from build123d import *

# Parameters (mm, degrees)
F1_DEPTH = 800
F2_R     = 10
F3_R     = 0.2


with BuildPart() as f1:
    # F0 (on Right) → F1 (new body)
    with BuildSketch(Plane.YZ):
        Polygon((100.824344, 4.7625), (125.181556, 0), (150, 0), (2.787639, 28.784037), (1.873746, 24.110044), (6.636246, 23.178845), align=None)
        Polygon((0, 4.7625), (0, 0), (125.181556, 0), (100.824344, 4.7625), (6.636246, 4.7625), (1.873746, 4.7625), align=None)
        Polygon((1.873746, 24.110044), (1.873746, 4.7625), (6.636246, 4.7625), (6.636246, 23.178845), align=None)
        Polygon((1.873746, 24.110044), (2.787639, 28.784037), (-8.682065, 26.173362), (-5.835444, 22.355227), align=None)
        Polygon((-10.756327, 4.761424), (0, 0), (0, 4.7625), (-7.229277, 7.963836), align=None)
        Polygon((-14.458972, 15.926554), (-10.756327, 4.761424), (-7.229277, 7.963836), (-9.718587, 15.468123), align=None)
        Polygon((-8.682065, 26.173362), (-14.458972, 15.926554), (-9.718587, 15.468123), (-5.835444, 22.355227), align=None)
    extrude(amount=F1_DEPTH)

    # F2
    f2_edges = [f1.edges().sort_by_distance(p)[0] for p in [
        (400, -8.682065, 26.173362),
        (400, -14.458972, 15.926554),
        (400, 2.787639, 28.784037),
        (400, -10.756327, 4.761424),
        (400, 0, 0),
    ]]
    fillet(f2_edges, radius=F2_R)

    # F3
    f3_edges = [f1.edges().sort_by_distance(p)[0] for p in [
        (400, 150, 0),
    ]]
    fillet(f3_edges, radius=F3_R)


solid = f1.part
The listing builds one solid part. Answer for the finished solid, in the listing's coordinates (mm). A direction names the side the tool comes from. Coordinates: 2 decimals unless noted, no trailing zeros. Loops run counter-clockwise (first coordinate to the right, second up) from the corner with the lowest first, then second, coordinate; pieces in that order, holes last.
1) Flat-ended cylindrical pins translate along their axes: pin 1 Ø0.9 at (x, y) = (530, 0.5) entering from +Z; pin 2 Ø6 at (x, z) = (338.5, 10.5) entering from -Y; pin 3 Ø8 at (x, y) = (249, 38) entering from +Z. Find the tip coordinate at first contact, or state that the pin passes through.
2) Determine the mould class of faces 3 (the face through (800, 55, 4)), 4 (the face through (394.4, 53.07, 14.1)), 5 (the face through (394.4, 77.42, 14.19)) for opening direction Y: pulls with the +Y half, pulls with the -Y half, needs draft (parallel to the pull), parting line crosses it, or undercut.
3) Find section B-B on y = 58. Write down the section's boundary in (x, z).
4) Find section C-C on y = 127. Write down the section's boundary in (x, z), then the cut area to 3 significant figures.
5) Find the intervals of material crossed by L1, parallel to Z at x = 607.5, y = 104; L2, parallel to Z at x = 279.5, y = 55.5; L3, parallel to Z at x = 160.5, y = 105, in increasing order.
6) A tool of negligible diameter and unlimited length cuts with its end or side. For faces 1 (the face through (394, 1.874, 15)), 2 (the face through (0, 55, 4)), from which of +Z, -Z, +X, -X, +Y, -Y can it reach the whole face along a straight path? Write none if from no direction.
7) Find section A-A on x = 100. Write down the section's boundary in (y, z).
Values:
1. pin 1: stops at z = 28.36
1. pin 2: stops at y = -13.48
1. pin 3: stops at z = 22.68
2. face 3: needs draft
2. face 4: undercut
2. face 5: pulls with the +Y half
3. outline: (0, 0) - (800, 0) - (800, 4.76) - (0, 4.76) - close; (0, 13.14) - (800, 13.14) - (800, 17.99) - (0, 17.99) - close
4. outline: (0, 0) - (800, 0) - (800, 4.5) - (0, 4.5) - close
4. area: 3,600 mm2
5. L1: z = 0 to 8.99
5. L2: z = 0 to 4.76, 13.62 to 18.48
5. L3: z = 0 to 8.8
6. face 1: +X, -X
6. face 2: +Z, -Z, -X, +Y, -Y
7. outline: (-13.07, 11.72) - (-12.15, 8.97) arc R10 ccw to (-6.71, 2.97) - (-1.93, 0.86) arc R10 ccw to (2.11, 0) - (147.93, 0) arc R0.2 ccw to (147.97, 0.4) - (4.86, 28.38) arc R10 ccw to (0.73, 28.31) - (-4.36, 27.16) arc R10 ccw to (-10.86, 22.32) - (-12.28, 19.78) arc R10 ccw to start; hole (-9.72, 15.47) - (-7.23, 7.96) - (0, 4.76) - (1.87, 4.76) - (1.87, 24.11) - (-5.84, 22.36) - close; hole (6.64, 4.76) - (100.82, 4.76) - (6.64, 23.18) - close
